Autodesk Inventor part; units mm, degrees
ref_plane "YZ Plane" through (0, 0, 0) normal (1, 0, 0) x (0, 1, 0)
ref_plane "XZ Plane" through (0, 0, 0) normal (0, 1, 0) x (-1, 0, 0)
ref_plane "XY Plane" through (0, 0, 0) normal (0, 0, 1) x (1, 0, 0)
sketch "Эскиз1" plane through (0, 0, 0) normal (0, 1, 0) x (-1, 0, 0)
  line L0 (10.55, 0) -> (5.275, -9.1366)
  line L1 (5.275, -9.1366) -> (-5.275, -9.1366)
  line L2 (-5.275, -9.1366) -> (-10.55, 0)
  line L3 (-10.55, 0) -> (-5.275, 9.1366)
  line L4 (-5.275, 9.1366) -> (5.275, 9.1366)
  line L5 (5.275, 9.1366) -> (10.55, 0)
  circle A0 centre (0, 0) radius 6
  dimension "d0" = 21.1
  dimension "d1" = 12
extrude "Выдавливание1" add sketch "Эскиз1" along normal blind 10
thread "Резьба1"
properties part number "KB33-046-002-003 - Фиксирующая гайка"
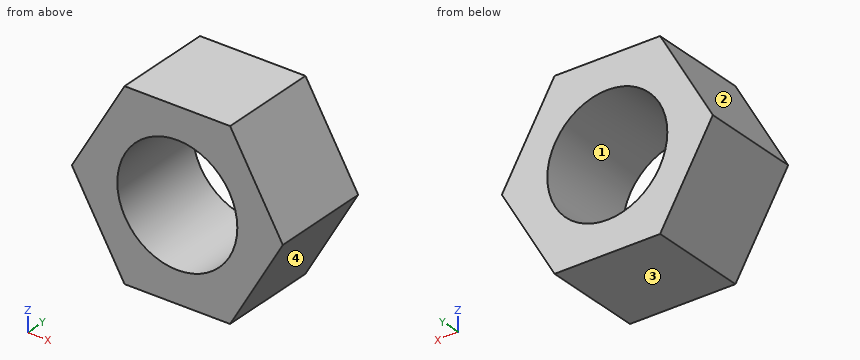
Check sheet for the modelled part. Datum: model origin and axes. Units: mm. Face numbers are marked on the shaded views. Give positions to 0.01 mm unless a question says otherwise; leave off trailing zeros. Write each loop counter-clockwise with the first axis right and the second up, starting at its lowest first coordinate (ties: lowest second). Pieces come first, ordered by that corner, then holes.
Item 1: Cross-section at B-B (y = 8). Enter the section's corners in (x, z) (3 decimals).
Item 2: Scan lines: L1, parallel to Z at x = 0, y = 6; L2, parallel to X at y = 9.5, z = -1; L3, parallel to Z at x = 4.25, y = 7.25. Record each from-to range of solid material in increasing order.
Item 3: Cross-section at A-A (x = 0). Enter the section's corners in (y, z).
Item 4: Gauge pin test, flat ends, axial feed: pin 1 (1 mm diameter, centred on y = 4.5, z = 4.5, fed in from +X); pin 2 (4 mm diameter, centred on x = -2, z = -1.5, fed in from -Y); pin 3 (4 mm diameter, centred on x = -6, y = 1, fed in from -Z); pin 4 (5 mm diameter, centred on y = 8, z = 2, fed in from -X). Record the tip position at first contact, or that the pin passes through.
Item 5: Draft check along X on the marked faces 1, 2, 3 and 4. Enter one of: released by +X, released by -X, zero draft, split by the parting line, or undercut.
Item 6: Cross-section at C-C (z = 2.25). Enter the section's corners in (x, y), and give its area (3 significant figures).
Item 7: Cross-section at D-D (x = -6.5). Enter the section's corners in (y, z), and give its area (3 significant figures).
Report:
1. outline: (-10.55, 0) - (-5.275, -9.137) - (5.275, -9.137) - (10.55, 0) - (5.275, 9.137) - (-5.275, 9.137) - close; hole circle Ø12 at (0, 0)
2. L1: z = -9.14 to -6, 6 to 9.14
2. L2: x = -9.97 to -5.92, 5.92 to 9.97
2. L3: z = -9.14 to -4.24, 4.24 to 9.14
3. outline: (0, -9.14) - (10, -9.14) - (10, -6) - (0, -6) - close; (0, 6) - (10, 6) - (10, 9.14) - (0, 9.14) - close
4. pin 1: stops at x = 8.24
4. pin 2: passes through
4. pin 3: stops at z = -9.14
4. pin 4: stops at x = -10.55
5. face 1: undercut
5. face 2: released by -X
5. face 3: zero draft
5. face 4: released by +X
6. outline: (-9.25, 0) - (-5.56, 0) - (-5.56, 10) - (-9.25, 10) - close; (5.56, 0) - (9.25, 0) - (9.25, 10) - (5.56, 10) - close
6. area: 73.8 mm2
7. outline: (0, -7.01) - (10, -7.01) - (10, 7.01) - (0, 7.01) - close
7. area: 140 mm2
